Model file for the job. Use its own axes, mm. Round coordinates to 2 decimals unless told otherwise and drop trailing zeros. Order: outer loops, then holes, each group sorted by start corner. A loop starts at its lowest first (then second) coordinate and runs counter-clockwise, first axis right, second up. Notation, with made-up numbers: M 56.25,76 L 113.25,76 A32 ccw 113.25,113 Z; hole C 83,-3 d9. An arc over 180 degrees is marked long. Return JSON: item names as keys, results as strings. Group by question number.
Item 1: Slice it at C-C on y = -9.5. Write the cut outline in (x, z) (3 decimals), then the cut area to 3 significant figures.
Item 2: Slice it at A-A on x = 0. Write the cut outline in (y, z).
Item 3: Pin check, flat tips, straight feed: pin 1 Ø1.1 at (y, z) = (15, 0.5) entering from +X; pin 2 Ø2 at (x, z) = (-8, 1) entering from -Y; pin 3 Ø11 at (x, y) = (-5, -8.5) entering from -Z. Stop position of each tip, or through.
Item 4: Slice it at B-B on y = 0. Write the cut outline in (x, z).
Item 5: Pull direction X, two halves, no side cores. Call faces 1 (the face through (-4, -15, 1)), 2 (the face through (22, 0, -3)), 3 (the face through (12, 17, -1.5)), 4 (the face through (2.502, 18.067, -0.073)): pulls with the +X half, pulls with the -X half, needs draft (parallel to the pull), parting line crosses it, or undercut.
Item 6: Probe line 1 along Y through (x, z) = (-5.5, 2); line 2 along Y through (x, z) = (2.5, -2); line 3 along X through (y, z) = (3, 0.25). List the from-to ranges inside material, lowest first.
Item 7: Slice it at D-D on x = 15. Write the cut outline in (y, z).
from build123d import *

# Parameters (mm, degrees)
SKETCH_1_R               = 17.4
EXTRUDE_1_DEPTH          = 5.6
SKETCH_2_R               = 1.7
CUT_EXTRUDE_1_DEPTH      = 26.23648153
SKETCH_3_R               = 7
CUT_EXTRUDE_2_DEPTH      = 26.23648153
SKETCH_4_R               = 2.8
CUT_EXTRUDE_3_DEPTH      = 3
SKETCH_5_R               = 1.7
CUT_EXTRUDE_4_DEPTH      = 26.23648153
CUT_EXTRUDE_5_DEPTH      = 2.5
SKETCH_7_W               = 16.1
SKETCH_7_H               = 16.1
CUT_EXTRUDE_6_DEPTH      = 1.5
CHAMFER_1_SIZE           = 0.5
SKETCH_9_W               = 2.2
SKETCH_9_H               = 8
SKETCH_9_W_2             = 8
SKETCH_9_H_2             = 2.2
CUT_EXTRUDE_7_DEPTH      = 26.281613873
BOSS_EXTRUDE1_DEPTH      = 5.6
BOSS_EXTRUDE1_DEPTH_BACK = 4
SKETCH1_R                = 20.65
SKETCH1_R_2              = 17.4
SKETCH3_R                = 23
SKETCH3_R_2              = 20.65
BOSS_EXTRUDE2_DEPTH      = 2.5
SKETCH4_R                = 18
CUT_EXTRUDE3_DEPTH       = 4
SKETCH5_W                = 1
SKETCH5_H                = 8
CUT_EXTRUDE4_DEPTH       = 10
CUT_EXTRUDE6_DEPTH       = 10
FILLET3_R                = 1
CUT_EXTRUDE7_START       = -3.1
SKETCH10_R               = 23
CUT_EXTRUDE7_DEPTH       = 3.1


with BuildPart() as part:
    # 草图1 → 凸台-拉伸1 (new body)
    with BuildSketch(Plane.XY):
        Circle(SKETCH_1_R)
    extrude(amount=EXTRUDE_1_DEPTH)

    # 草图2 → 切除-拉伸1 (cut, through all)
    with BuildSketch(Plane.XY.offset(5.6)):
        with Locations((-6.717514421, 6.717514421)):
            Circle(SKETCH_2_R)
        with Locations((6.717514421, -6.717514421)):
            Circle(SKETCH_2_R)
    extrude(amount=-CUT_EXTRUDE_1_DEPTH, mode=Mode.SUBTRACT)

    # 草图3 → 切除-拉伸2 (cut, through all)
    with BuildSketch(Plane.XY.offset(5.6)):
        Circle(SKETCH_3_R)
    extrude(amount=-CUT_EXTRUDE_2_DEPTH, mode=Mode.SUBTRACT)

    # 草图4 → 切除-拉伸3 (cut)
    with BuildSketch(Plane.XY.offset(5.6)):
        with Locations((-6.717514421, 6.717514421)):
            Circle(SKETCH_4_R)
        with Locations((6.717514421, -6.717514421)):
            Circle(SKETCH_4_R)
    extrude(amount=-CUT_EXTRUDE_3_DEPTH, mode=Mode.SUBTRACT)

    # 草图5 → 切除-拉伸4 (cut, through all)
    with BuildSketch(Plane.XY.offset(5.6)):
        with Locations((8.05, 8)):
            Circle(SKETCH_5_R)
        with Locations((-8.05, -8)):
            Circle(SKETCH_5_R)
    extrude(amount=-CUT_EXTRUDE_4_DEPTH, mode=Mode.SUBTRACT)

    # 草图6 → 切除-拉伸5 (cut)
    with BuildSketch(Plane(origin=(0, 0, 0), x_dir=(-1, 0, 0), z_dir=(0, 0, -1))):
        Polygon((4.766838493, -8), (6.408419246, -10.84330127), (9.691580754, -10.84330127), (11.333161507, -8), (9.691580754, -5.15669873), (6.408419246, -5.15669873), align=None)
        Polygon((-4.766838493, 8), (-6.408419246, 10.84330127), (-9.691580754, 10.84330127), (-11.333161507, 8), (-9.691580754, 5.15669873), (-6.408419246, 5.15669873), align=None)
    extrude(amount=-CUT_EXTRUDE_5_DEPTH, mode=Mode.SUBTRACT)

    # 草图7 → 切除-拉伸6 (cut)
    with BuildSketch(Plane.XY.offset(5.6)):
        Rectangle(SKETCH_7_W, SKETCH_7_H)
    extrude(amount=-CUT_EXTRUDE_6_DEPTH, mode=Mode.SUBTRACT)

    # 倒角1
    chamfer_1_edges = [part.edges().sort_by_distance(p)[0] for p in [
        (8.05, 1.022551258, 5.6),
        (1.047918985, 8.05, 5.6),
        (-8.05, -1.022551258, 5.6),
        (-1.047918985, -8.05, 5.6),
    ]]
    chamfer(chamfer_1_edges, length=CHAMFER_1_SIZE)

    # 草图8 → 旋转1 (revolve)
    with BuildSketch(Plane(origin=(0, 0, 0), x_dir=(0, 0, -1), z_dir=(1, 0, 0)), mode=Mode.PRIVATE) as revolve_1_sk:
        Polygon((0, 17.4), (0, 17.2), (0.2, 17.4), align=None)
    revolve(revolve_1_sk.sketch.rotate(Axis((0, 0, 0), (0, 0, 1)), 90), axis=Axis((0, 0, 0), (0, 0, 1)))

    # 草图9 → 切除-拉伸7 (cut, through all)
    with BuildSketch(Plane.XY.offset(5.6)):
        with Locations((14.6, 0)):
            Rectangle(SKETCH_9_W, SKETCH_9_H)
        with Locations((0, 14.6)):
            Rectangle(SKETCH_9_W_2, SKETCH_9_H_2)
        with Locations((-14.6, 0)):
            Rectangle(SKETCH_9_W, SKETCH_9_H)
        with Locations((0, -14.6)):
            Rectangle(SKETCH_9_W_2, SKETCH_9_H_2)
    extrude(amount=-CUT_EXTRUDE_7_DEPTH, mode=Mode.SUBTRACT)

    # Sketch1 → Boss-Extrude1 (add, two sides: drawn at the far end of the back side and taken through both)
    with BuildSketch(Plane.XY.offset(-BOSS_EXTRUDE1_DEPTH_BACK)):
        Circle(SKETCH1_R)
        Circle(SKETCH1_R_2, mode=Mode.SUBTRACT)
    extrude(amount=BOSS_EXTRUDE1_DEPTH + BOSS_EXTRUDE1_DEPTH_BACK)

    # Sketch3 → Boss-Extrude2 (add)
    with BuildSketch(Plane(origin=(0, 0, -4), x_dir=(-1, 0, 0), z_dir=(0, 0, -1))):
        Circle(SKETCH3_R)
        with Locations(Location((0, 0, 0), (0, 0, 180))):
            Circle(SKETCH3_R_2, mode=Mode.SUBTRACT)
    extrude(amount=-BOSS_EXTRUDE2_DEPTH)

    # Sketch4 → Cut-Extrude3 (cut)
    with BuildSketch(Plane(origin=(0, 0, -4), x_dir=(-1, 0, 0), z_dir=(0, 0, -1))):
        Circle(SKETCH4_R)
    extrude(amount=-CUT_EXTRUDE3_DEPTH, mode=Mode.SUBTRACT)

    # Sketch5 → Cut-Extrude4 (cut)
    with BuildSketch(Plane(origin=(0, 0, -4), x_dir=(-1, 0, 0), z_dir=(0, 0, -1))):
        with Locations((22.5, 0)):
            Rectangle(SKETCH5_W, SKETCH5_H)
        with Locations((-22.5, 0)):
            Rectangle(SKETCH5_W, SKETCH5_H)
    extrude(amount=-CUT_EXTRUDE4_DEPTH, mode=Mode.SUBTRACT)

    # Sketch7 → Cut-Extrude6 (cut)
    with BuildSketch(Plane(origin=(0, 0, -4), x_dir=(-1, 0, 0), z_dir=(0, 0, -1))):
        with BuildLine():
            Line((0, 18), (0, 22.3))
            Line((0, 22.3), (-2.6, 22.3))
            Line((-2.6, 22.3), (-2.6, 17.811232411))
            ThreePointArc((-2.6, 17.811232411), (-1.303421766, 17.952746077), (0, 18))
        make_face()
        with BuildLine():
            Line((0, 17.5), (0, 18))
            ThreePointArc((0, 18), (-1.303421766, 17.952746077), (-2.6, 17.811232411))
            Line((-2.6, 17.811232411), (-2.6, 17.5))
            Line((-2.6, 17.5), (0, 17.5))
        make_face()
        with BuildLine():
            Line((2.6, 22.3), (0, 22.3))
            Line((0, 22.3), (0, 18))
            ThreePointArc((0, 18), (1.303421766, 17.952746077), (2.6, 17.811232411))
            Line((2.6, 17.811232411), (2.6, 22.3))
        make_face()
        with BuildLine():
            ThreePointArc((2.6, 17.811232411), (1.303421766, 17.952746077), (0, 18))
            Line((0, 18), (0, 17.5))
            Line((0, 17.5), (2.6, 17.5))
            Line((2.6, 17.5), (2.6, 17.811232411))
        make_face()
    extrude(amount=-CUT_EXTRUDE6_DEPTH, mode=Mode.SUBTRACT)

    # Fillet3
    # the kernel refuses this fillet: 1 mm, written as the material it adds along each edge
    with BuildSketch(Plane(origin=(2.6, 22.3, -4), x_dir=(-1, 0, 0), z_dir=(0, 0, 1))) as fillet3_piece_1:
        with BuildLine():
            CenterArc((FILLET3_R, FILLET3_R), FILLET3_R, 180, 90)
            Line((0, FILLET3_R), (-FILLET3_R * 0.02, FILLET3_R))
            Line((-FILLET3_R * 0.02, FILLET3_R), (-FILLET3_R * 0.02, -FILLET3_R * 0.02))
            Line((-FILLET3_R * 0.02, -FILLET3_R * 0.02), (FILLET3_R, -FILLET3_R * 0.02))
            Line((FILLET3_R, -FILLET3_R * 0.02), (FILLET3_R, 0))
        make_face()
    extrude(amount=2.5)
    with BuildSketch(Plane(origin=(-2.6, 22.3, -4), x_dir=(1, 0, 0), z_dir=(0, 0, 1))) as fillet3_piece_2:
        with BuildLine():
            CenterArc((FILLET3_R, -FILLET3_R), FILLET3_R, 90, 90)
            Line((0, -FILLET3_R), (-FILLET3_R * 0.02, -FILLET3_R))
            Line((-FILLET3_R * 0.02, -FILLET3_R), (-FILLET3_R * 0.02, FILLET3_R * 0.02))
            Line((-FILLET3_R * 0.02, FILLET3_R * 0.02), (FILLET3_R, FILLET3_R * 0.02))
            Line((FILLET3_R, FILLET3_R * 0.02), (FILLET3_R, 0))
        make_face()
    extrude(amount=2.5)
    with BuildSketch(Plane(origin=(-2.6, 17.5, -6), x_dir=(0, 1, 0), z_dir=(0, 0, 1))) as fillet3_piece_3_section:
        with BuildLine():
            CenterArc((FILLET3_R, -FILLET3_R), FILLET3_R, 90, 90)
            Line((0, -FILLET3_R), (-FILLET3_R * 0.02, -FILLET3_R))
            Line((-FILLET3_R * 0.02, -FILLET3_R), (-FILLET3_R * 0.02, FILLET3_R * 0.02))
            Line((-FILLET3_R * 0.02, FILLET3_R * 0.02), (FILLET3_R, FILLET3_R * 0.02))
            Line((FILLET3_R, FILLET3_R * 0.02), (FILLET3_R, 0))
        make_face()
    fillet3_piece_3 = extrude(amount=11.6, mode=Mode.PRIVATE)
    fillet3_piece_3 = split(fillet3_piece_3, bisect_by=Plane(origin=(-2.544482942, 18.024809788, 0), z_dir=(0, 0, -1)), keep=Keep.TOP, mode=Mode.PRIVATE)
    fillet3_piece_3 = fillet3_piece_3 - Plane(origin=(0, 0, -2), x_dir=(-1, 0, 0), z_dir=(0, 0, -1)) * Cylinder(18, 28, mode=Mode.PRIVATE)
    fillet3_piece_3 = split(fillet3_piece_3, bisect_by=Plane(origin=(-2.544482942, 18.024809788, -4), z_dir=(0, 0, 1)), keep=Keep.TOP, mode=Mode.PRIVATE)
    add(fillet3_piece_3)
    with BuildSketch(Plane(origin=(-2.6, 17.5, 0), x_dir=(0, 1, 0), z_dir=(0, 0, 1))) as fillet3_piece_4_section:
        with BuildLine():
            CenterArc((FILLET3_R, -FILLET3_R), FILLET3_R, 90, 90)
            Line((0, -FILLET3_R), (-FILLET3_R * 0.02, -FILLET3_R))
            Line((-FILLET3_R * 0.02, -FILLET3_R), (-FILLET3_R * 0.02, FILLET3_R * 0.02))
            Line((-FILLET3_R * 0.02, FILLET3_R * 0.02), (FILLET3_R, FILLET3_R * 0.02))
            Line((FILLET3_R, FILLET3_R * 0.02), (FILLET3_R, 0))
        make_face()
    fillet3_piece_4 = extrude(amount=5.6, mode=Mode.PRIVATE)
    fillet3_piece_4 = fillet3_piece_4 - Plane(origin=(0, 0, 2.8), x_dir=(-1, 0, 0), z_dir=(0, 0, -1)) * Cylinder(18, 16, mode=Mode.PRIVATE)
    add(fillet3_piece_4)
    with BuildSketch(Plane(origin=(-2.6, 17.5, 0), x_dir=(0, 1, 0), z_dir=(0, 0, 1))) as fillet3_piece_5_section:
        with BuildLine():
            CenterArc((FILLET3_R, -FILLET3_R), FILLET3_R, 90, 90)
            Line((0, -FILLET3_R), (-FILLET3_R * 0.02, -FILLET3_R))
            Line((-FILLET3_R * 0.02, -FILLET3_R), (-FILLET3_R * 0.02, FILLET3_R * 0.02))
            Line((-FILLET3_R * 0.02, FILLET3_R * 0.02), (FILLET3_R, FILLET3_R * 0.02))
            Line((FILLET3_R, FILLET3_R * 0.02), (FILLET3_R, 0))
        make_face()
    fillet3_piece_5 = extrude(amount=5.6, mode=Mode.PRIVATE)
    fillet3_piece_5 = fillet3_piece_5 & Plane(origin=(0, 0, 2.8), x_dir=(-1, 0, 0), z_dir=(0, 0, -1)) * Cylinder(18, 16, mode=Mode.PRIVATE)
    add(fillet3_piece_5)
    with BuildSketch(Plane(origin=(2.6, 17.5, -6), x_dir=(-1, 0, 0), z_dir=(0, 0, 1))) as fillet3_piece_6_section:
        with BuildLine():
            CenterArc((FILLET3_R, -FILLET3_R), FILLET3_R, 90, 90)
            Line((0, -FILLET3_R), (-FILLET3_R * 0.02, -FILLET3_R))
            Line((-FILLET3_R * 0.02, -FILLET3_R), (-FILLET3_R * 0.02, FILLET3_R * 0.02))
            Line((-FILLET3_R * 0.02, FILLET3_R * 0.02), (FILLET3_R, FILLET3_R * 0.02))
            Line((FILLET3_R, FILLET3_R * 0.02), (FILLET3_R, 0))
        make_face()
    fillet3_piece_6 = extrude(amount=11.6, mode=Mode.PRIVATE)
    fillet3_piece_6 = split(fillet3_piece_6, bisect_by=Plane(origin=(2.544482942, 18.024809788, 0), z_dir=(0, 0, -1)), keep=Keep.TOP, mode=Mode.PRIVATE)
    fillet3_piece_6 = fillet3_piece_6 - Plane(origin=(0, 0, -2), x_dir=(-1, 0, 0), z_dir=(0, 0, -1)) * Cylinder(18, 28, mode=Mode.PRIVATE)
    fillet3_piece_6 = split(fillet3_piece_6, bisect_by=Plane(origin=(2.544482942, 18.024809788, -4), z_dir=(0, 0, 1)), keep=Keep.TOP, mode=Mode.PRIVATE)
    add(fillet3_piece_6)
    with BuildSketch(Plane(origin=(2.6, 17.5, 0), x_dir=(-1, 0, 0), z_dir=(0, 0, 1))) as fillet3_piece_7_section:
        with BuildLine():
            CenterArc((FILLET3_R, -FILLET3_R), FILLET3_R, 90, 90)
            Line((0, -FILLET3_R), (-FILLET3_R * 0.02, -FILLET3_R))
            Line((-FILLET3_R * 0.02, -FILLET3_R), (-FILLET3_R * 0.02, FILLET3_R * 0.02))
            Line((-FILLET3_R * 0.02, FILLET3_R * 0.02), (FILLET3_R, FILLET3_R * 0.02))
            Line((FILLET3_R, FILLET3_R * 0.02), (FILLET3_R, 0))
        make_face()
    fillet3_piece_7 = extrude(amount=5.6, mode=Mode.PRIVATE)
    fillet3_piece_7 = fillet3_piece_7 & Plane(origin=(0, 0, 2.8), x_dir=(-1, 0, 0), z_dir=(0, 0, -1)) * Cylinder(18, 16, mode=Mode.PRIVATE)
    add(fillet3_piece_7)
    with BuildSketch(Plane(origin=(2.6, 17.5, 0), x_dir=(-1, 0, 0), z_dir=(0, 0, 1))) as fillet3_piece_8_section:
        with BuildLine():
            CenterArc((FILLET3_R, -FILLET3_R), FILLET3_R, 90, 90)
            Line((0, -FILLET3_R), (-FILLET3_R * 0.02, -FILLET3_R))
            Line((-FILLET3_R * 0.02, -FILLET3_R), (-FILLET3_R * 0.02, FILLET3_R * 0.02))
            Line((-FILLET3_R * 0.02, FILLET3_R * 0.02), (FILLET3_R, FILLET3_R * 0.02))
            Line((FILLET3_R, FILLET3_R * 0.02), (FILLET3_R, 0))
        make_face()
    fillet3_piece_8 = extrude(amount=5.6, mode=Mode.PRIVATE)
    fillet3_piece_8 = fillet3_piece_8 - Plane(origin=(0, 0, 2.8), x_dir=(-1, 0, 0), z_dir=(0, 0, -1)) * Cylinder(18, 16, mode=Mode.PRIVATE)
    add(fillet3_piece_8)

    # Sketch10 → Cut-Extrude7 (cut)
    with BuildSketch(Plane.XY.offset(5.6).offset(CUT_EXTRUDE7_START)):
        Circle(SKETCH10_R)
    extrude(amount=CUT_EXTRUDE7_DEPTH, mode=Mode.SUBTRACT)


solid = part.part
Output values:
{
 "1": {"outline": "M -20.946,-4 L -15.289,-4 L -15.289,0 L -10.467,0 L -10.467,2.5 L -18.335,2.5 L -18.335,-1.5 L -20.946,-1.5 Z; M -5.633,0 L 15.289,0 L 15.289,-4 L 20.946,-4 L 20.946,-1.5 L 18.335,-1.5 L 18.335,2.5 L -5.633,2.5 Z", "area": "117 mm²"},
 "2": {"outline": "M -23,-4 L -18,-4 L -18,0 L -15.7,0 L -15.7,2.5 L -20.65,2.5 L -20.65,-1.5 L -23,-1.5 Z; M -13.5,0 L -7,0 L -7,2.5 L -13.5,2.5 Z; M 7,0 L 13.5,0 L 13.5,2.5 L 7,2.5 Z; M 15.7,0 L 17.5,0 L 17.5,2.5 L 15.7,2.5 Z; M 22.3,-4 L 23,-4 L 23,-1.5 L 22.3,-1.5 Z"},
 "3": {"pin 1": "x = 14.75", "pin 2": "y = -19.43", "pin 3": "z = 0"},
 "4": {"outline": "M -22,-4 L -18,-4 L -18,0 L -15.7,0 L -15.7,2.5 L -20.65,2.5 L -20.65,-1.5 L -22,-1.5 Z; M -13.5,0 L -7,0 L -7,2.5 L -13.5,2.5 Z; M 7,0 L 13.5,0 L 13.5,2.5 L 7,2.5 Z; M 15.7,0 L 18,0 L 18,-4 L 22,-4 L 22,-1.5 L 20.65,-1.5 L 20.65,2.5 L 15.7,2.5 Z"},
 "5": {"face 1": "undercut", "face 2": "pulls with the +X half", "face 3": "needs draft", "face 4": "undercut"},
 "6": {"line 1": "-19.9 to -9.27, -6.73 to -4.33, 4.33 to 5.53, 7.9 to 19.9", "line 2": "-22.86 to -17.83, 17.83 to 18.06, 21.74 to 22.86", "line 3": "-20.43 to -15.7, -13.5 to -6.32, 6.32 to 13.5, 15.7 to 20.43"},
 "7": {"outline": "M -17.44,-4 L -9.95,-4 L -9.95,0 L -4,0 L -4,2.5 L -14.19,2.5 L -14.19,-1.5 L -17.44,-1.5 Z; M 4,0 L 9.95,0 L 9.95,-4 L 17.44,-4 L 17.44,-1.5 L 14.19,-1.5 L 14.19,2.5 L 4,2.5 Z"}
}
